The model under review builds one solid part; all positions refer to its coordinate system, in mm. A direction names the side the tool comes from. Give positions to 0.01 mm unless a question says otherwise; leave off trailing zeros. Loops run counter-clockwise (first coordinate to the right, second up) from the corner with the lowest first, then second, coordinate; pieces in that order, holes last. Notation, with made-up numbers: M -26,-6 L 16,-6 A22 ccw 16,21 Z; hole C 65,74.5 d1. An arc over 180 degrees is marked long. Put each result on its own line as item: value. Start each with the question number.
```python
from build123d import *

# Parameters (mm, degrees)
F1_DEPTH = 55
F2_W     = 15
F2_H     = 25
F3_DEPTH = 57.6
F4_R     = 5
F5_DEPTH = 30


with BuildPart() as f1:
    # F0 (on Front) → F1 (new body)
    with BuildSketch(Plane.XZ):
        Polygon((-37.5, 30), (-37.5, 0), (-15, 0), (-15, -30), (0, -30), (15, -30), (15, 0), (37.5, 0), (37.5, 30), (0, 30), align=None)
    extrude(amount=-F1_DEPTH)

    # F2 (on face) → F3 (cut)
    with BuildSketch(Plane.XY.offset(30)):
        with Locations((-30, 42.5)):
            Rectangle(F2_W, F2_H)
        with Locations((30, 42.5)):
            Rectangle(F2_W, F2_H)
    extrude(amount=-F3_DEPTH, mode=Mode.SUBTRACT)

    # F4 (on face) → F5 (join)
    with BuildSketch(Plane.XY.offset(30)):
        with BuildLine():
            Line((-14.5, 0), (-37.5, 0))
            Line((-37.5, 0), (-37.5, -15))
            ThreePointArc((-37.5, -15), (-26, -26.5), (-14.5, -15))
            Line((-14.5, -15), (-14.5, 0))
        make_face()
        with Locations((-26, -15)):
            Circle(F4_R, mode=Mode.SUBTRACT)
        with BuildLine():
            Line((37.5, 0), (14.5, 0))
            Line((14.5, 0), (14.5, -15))
            ThreePointArc((14.5, -15), (26, -26.5), (37.5, -15))
            Line((37.5, -15), (37.5, 0))
        make_face()
        with Locations((26, -15)):
            Circle(F4_R, mode=Mode.SUBTRACT)
    extrude(amount=-F5_DEPTH)


solid = f1.part
```
Item 1: Consider section B-B, the plane z = 16.5. Write out the cut boundary in (x, y).
Item 2: Consider section D-D, the plane y = 33. Write out the cut boundary in (x, z).
Item 3: Tool access review of faces 5 (the flat face through (-1, 15, 30)), 6 (the flat face through (-22.5, 42, 15)), 7 (the flat face through (14.5, -7, 15)), 8 (the flat face through (15, 27, -15)), 9 (the flat face through (30, 30, 15)): name each direction out of +Z, -Z, +X, -X, +Y, -Y from which nothing blocks a thin tool from reaching the whole face with its end or side.
Item 4: Clearance check with flat-ended pins moving along their axes: pin 1 Ø7.5 at (x, z) = (29, 9) entering from +Y; pin 2 Ø15 at (y, z) = (30.5, -18.5) entering from +X; pin 3 Ø18.5 at (x, y) = (29.5, 0.5) entering from -Z. State where each tip first meets the part, or that it passes through.
Item 5: Consider section C-C, the plane y = -5.5. Write out the cut boundary in (x, z).
Item 6: Draft analysis for pull direction X (two halves, no side actions). For faces 1 (the flat face through (0, 27, -30)), 2 (the cylindrical face through (-26.253, -26.497, 15.21)), 3 (the flat face through (-37.5, 8, 15)), 4 (the cylindrical face through (22, -18, 15)), state which applies: +X half, -X half, draft (parallel to the pull), parting line (faces both ways), or undercut.
Item 7: To check wall thickness, follow L1, parallel to Y at x = -26, z = 8.75; L2, parallel to Z at x = 16, y = 45; L3, parallel to Y at x = 3, z = 26. State the ranges of each line that lie inside material, in increasing order. Write a range as [from, to].
Item 8: Consider section A-A, the plane x = -26. Write out the cut boundary in (y, z), plus the area to 4 significant figures.
Report:
1. outline: M -37.5,-15 A11.5 ccw -14.5,-15 L -14.5,0 L 14.5,0 L 14.5,-15 A11.5 ccw 37.5,-15 L 37.5,30 L 22.5,30 L 22.5,55 L -22.5,55 L -22.5,30 L -37.5,30 Z; hole C -26,-15 d10; hole C 26,-15 d10
2. outline: M -22.5,0 L -15,0 L -15,-30 L 15,-30 L 15,0 L 22.5,0 L 22.5,30 L -22.5,30 Z
3. face 5: +Z, +X, -X, +Y, -Y
3. face 6: +Z, -Z, -X, +Y
3. face 7: +Z, -Z, -Y
3. face 8: -Z, +X, +Y, -Y
3. face 9: +Z, -Z, +X, +Y
4. pin 1: y = 30
4. pin 2: x = 15
4. pin 3: z = 0
5. outline: M -37.5,0 L -14.5,0 L -14.5,30 L -37.5,30 Z; M 14.5,0 L 37.5,0 L 37.5,30 L 14.5,30 Z
6. face 1: draft
6. face 2: undercut
6. face 3: -X half
6. face 4: undercut
7. L1: [-26.5, -20], [-10, 30]
7. L2: [0, 30]
7. L3: [0, 55]
8. outline: M -26.5,0 L -20,0 L -20,30 L -26.5,30 Z; M -10,0 L 30,0 L 30,30 L -10,30 Z
8. area: 1,395 mm²
